Here's how the part is built. I have some questions about the finished solid (model axes, mm). Round coordinates to 2 decimals unless told otherwise and drop trailing zeros. Loops run counter-clockwise (first coordinate to the right, second up) from the corner with the lowest first, then second, coordinate; pieces in that order, holes last. Notation, with made-up numbers: (-19, 74.25) -> (-2, 74.25) arc R10 ccw to (-2, 92.25) -> close; hole circle Ø4 at (-9, 21). An arc over 180 degrees is marked (long way). Use CSV: the item, a comma, the result in double quotes. Start each with the question number.
Autodesk Inventor part; units mm, degrees
ref_plane "YZ Plane" through (0, 0, 0) normal (1, 0, 0) x (0, 1, 0)
ref_plane "XZ Plane" through (0, 0, 0) normal (0, 1, 0) x (-1, 0, 0)
ref_plane "XY Plane" through (0, 0, 0) normal (0, 0, 1) x (1, 0, 0)
sketch "Sketch1" plane through (0, 0, 0) normal (0, 1, 0) x (-1, 0, 0)
  line L0 (-90, -40) -> (90, -40)
  line L1 (90, -40) -> (90, 40)
  line L2 (90, 40) -> (-90, 40)
  line L3 (-90, 40) -> (-90, -40)
  line L4 (-90, -40) -> (90, 40) construction
  line L5 (90, -40) -> (-90, 40) construction
  line L6 (90, 40) -> (90, 20)
  line L7 (90, 20) -> (-28, 20)
  line L8 (-28, 20) -> (-28, -20)
  line L9 (-28, -20) -> (-68, -20)
  line L10 (-68, -20) -> (-68, 20)
  line L11 (-68, 20) -> (-28, 20)
  line L12 (90, -40) -> (-72, -40)
  line L13 (90, 40) -> (-72, 40)
  line L14 (-90, 0) -> (-90, 14)
  line L15 (-90, 14) -> (-72, 40)
  line L16 (-90, 0) -> (-90, -14)
  line L17 (-90, -14) -> (-72, -40)
  circle A0 centre (-68, 20) radius 2.6
  circle A1 centre (-68, -20) radius 2.6
  circle A2 centre (-28, -20) radius 2.6
  circle A3 centre (-28, 20) radius 2.6
  circle A4 centre (-68, 0) radius 4
  point P0 (0, 0)
  dimension "d0" = 180
  dimension "d1" = 80
  dimension "d2" = 20
  dimension "d3" = 118
  dimension "d4" = 40
  dimension "d5" = 40
  dimension "d6" = 162
  dimension "d7" = 162
  dimension "d8" = 14
  dimension "d9" = 14
  dimension "d10" = 5.2
  dimension "d11" = 5.2
  dimension "d12" = 5.2
  dimension "d13" = 5.2
  dimension "d14" = 8
extrude "Extrusion1" add sketch "Sketch1" along normal blind 2 contours L17 L3 L15 L2 L1 L0 | A3 L8 A2 L9 A1 L10 A4 A0 L11
properties part number "motorholder"
Q1. I want a section at B-B, the plane x = 28. List the corners of the cut face in (y, z) for me, then the cut area to 3 significant figures.
Q2. I want a section at D-D, the plane z = -20. List the corners of the cut face in (x, y) for me.
Q3. I want a section at C-C, the plane z = 0. List the corners of the cut face in (x, y) for me.
Q4. I want a section at A-A, the plane x = 68. List the corners of the cut face in (y, z) for me.
Q5. I need wall thicknesses on line 1 along Z through (x, y) = (68, 1.35); line 2 along Z through (x, y) = (28, 0.7); line 3 along X through (y, z) = (1.2, 0). Which ranges of each line are inside material? Lowest first, please.
Q6. If we mould it in two halves opening along Z, with no side actions, what happens to faces 1 (the flat face through (81, 1, 27)), 2 (the flat face through (1, 0, 1)), 3 (the cylindrical face through (64.305, 0.986, 1.532))? For each: pulls with the +Z half, pulls with the -Z half, needs draft (parallel to the pull), parting line crosses it, or undercut.
Q7. Will this pin go through, and if not, where does the flat tip stop? pin 1 Ø10.5 at (x, z) = (68, 0) entering from -Y.
Values found:
1,outline,"(0, -40) -> (2, -40) -> (2, -22.6) -> (0, -22.6) -> close; (0, -17.4) -> (2, -17.4) -> (2, 17.4) -> (0, 17.4) -> close; (0, 22.6) -> (2, 22.6) -> (2, 40) -> (0, 40) -> close"
1,area,"139 mm2"
2,outline,"(-90, 0) -> (25.4, 0) -> (25.4, 2) -> (-90, 2) -> close; (30.6, 0) -> (65.4, 0) -> (65.4, 2) -> (30.6, 2) -> close; (70.6, 0) -> (85.85, 0) -> (85.85, 2) -> (70.6, 2) -> close"
3,outline,"(-90, 0) -> (64, 0) -> (64, 2) -> (-90, 2) -> close; (72, 0) -> (90, 0) -> (90, 2) -> (72, 2) -> close"
4,outline,"(0, -40) -> (2, -40) -> (2, -22.6) -> (0, -22.6) -> close; (0, -17.4) -> (2, -17.4) -> (2, -4) -> (0, -4) -> close; (0, 4) -> (2, 4) -> (2, 17.4) -> (0, 17.4) -> close; (0, 22.6) -> (2, 22.6) -> (2, 40) -> (0, 40) -> close"
5,line 1,"-40 to -22.6, -17.4 to -4, 4 to 17.4, 22.6 to 40"
5,line 2,"-40 to -22.6, -17.4 to 17.4, 22.6 to 40"
5,line 3,"-90 to 64, 72 to 90"
6,face 1,"pulls with the +Z half"
6,face 2,"needs draft"
6,face 3,"undercut"
7,pin 1,"y = 0"
